CAD build for the part. Positions are in the model's coordinates, mm. Face numbers are marked on the shaded views. Round coordinates to 2 decimals unless told otherwise and drop trailing zeros. Order: outer loops, then holes, each group sorted by start corner. A loop starts at its lowest first (then second) coordinate and runs counter-clockwise, first axis right, second up. Notation, with made-up numbers: (-14, 10.5) - (0, 10.5) arc R13 ccw to (0, 16.5) - close; hole circle Ø9 at (-20.75, 36.25). An arc over 180 degrees is marked (long way). Use one line per item in the form item = value. Start each with the question number.
from build123d import *

# Parameters (mm, degrees)
SKETCH_W            = 205
SKETCH_H            = 115
PAD_DEPTH           = 1.5
SKETCH001_W         = 205
SKETCH001_H         = 115
SKETCH001_W_2       = 200
SKETCH001_H_2       = 110
PAD001_DEPTH        = 7
SKETCH004_W         = 20.8
SKETCH004_H         = 1.2
POCKET_DEPTH        = 1.501
POCKET_DEPTH_BACK   = 7.001
POCKET001_DEPTH     = 10.4
PAD007_DEPTH        = 28.857143
LINEARPATTERN_COUNT = 4
LINEARPATTERN_PITCH = 58.714286
FILLET_R            = 2
CHAMFER_SIZE        = 1


with BuildPart() as part:
    # Sketch → Pad (new body)
    with BuildSketch(Plane.XY):
        Rectangle(SKETCH_W, SKETCH_H)
    extrude(amount=-PAD_DEPTH)

    # Sketch001 → Pad001 (join)
    with BuildSketch(Plane.XY):
        Rectangle(SKETCH001_W, SKETCH001_H)
        Rectangle(SKETCH001_W_2, SKETCH001_H_2, mode=Mode.SUBTRACT)
    extrude(amount=PAD001_DEPTH)

    # Sketch004 → Pocket (cut, two sides)
    with BuildSketch(Plane.XY) as pocket_sk:
        with Locations((0, -56.9)):
            Rectangle(SKETCH004_W, SKETCH004_H)
    extrude(amount=-POCKET_DEPTH, mode=Mode.SUBTRACT)
    extrude(pocket_sk.sketch, amount=POCKET_DEPTH_BACK, mode=Mode.SUBTRACT)

    # Sketch005 → Pocket001 (cut, symmetric)
    with BuildSketch(Plane.YZ):
        Polygon((-56.3, -1.5), (-55.3, -0.6609), (-55.3, 0.3391), (-56.3, 1.178199), align=None)
    extrude(amount=POCKET001_DEPTH, both=True, mode=Mode.SUBTRACT)

    # Sketch008 → Pad007 (join)
    with BuildSketch(Plane.YZ.offset(-102.5)):
        with BuildLine():
            Line((57.5, 7), (57.8, 7.3))
            ThreePointArc((61.906969, 5.384889), (61.356546, 9.565769), (57.8, 7.3))
            Line((61.906969, 5.384889), (57.5, 1.687003))
            Line((57.5, 7), (57.5, 1.687003))
        make_face()
        with BuildLine():
            Line((59.41611, 8.183877), (60.3, 9.067767))
            Line((60.3, 9.067767), (61.183875, 8.183892))
            ThreePointArc((59.41611, 8.183877), (60.30001, 6.05), (61.183875, 8.183892))
        make_face(mode=Mode.SUBTRACT)
    pad007 = extrude(amount=PAD007_DEPTH)

    # LinearPattern: Pad007 ×4
    with Locations(*[(i * LINEARPATTERN_PITCH, 0, 0) for i in range(1, LINEARPATTERN_COUNT)]):
        add(pad007)

    # Fillet
    fillet_edges = [part.edges().sort_by_distance(p)[0] for p in [
        (102.5, -57.5, 2.75),
        (102.5, 57.5, 0.093501),
        (-102.5, 57.5, 0.093501),
        (-102.5, -57.5, 2.75),
    ]]
    fillet(fillet_edges, radius=FILLET_R)

    # Chamfer
    chamfer_edges = [part.edges().sort_by_distance(p)[0] for p in [
        (55.45, -57.5, -1.5),
    ]]
    chamfer(chamfer_edges, length=CHAMFER_SIZE)


solid = part.part
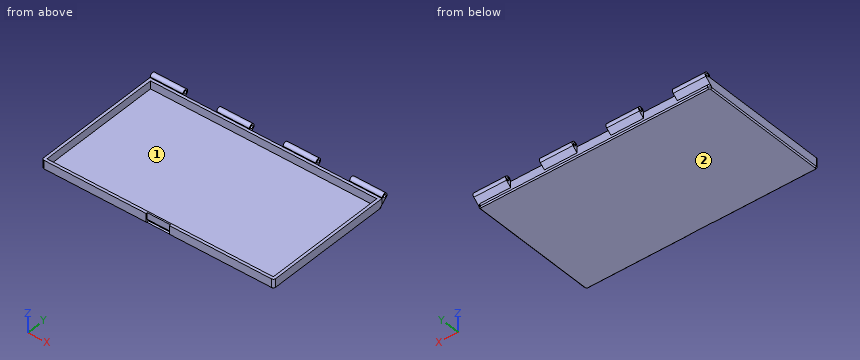
(1) Wall check: line 1 (Y direction, x = 45.5, z = 6); line 2 (X direction, y = 39, z = 3.25); line 3 (Z direction, x = 80.5, y = 54.5). Give the ranges that are in metal, low to high. Write a range as [from, to].
(2) Slice it at A-A (x = -62.5). Give the cut face in (y, z), and give its area (4 significant figures).
(3) Flat gauge pins, fed straight in: P1, Ø5.5, axis at x = 44, z = 2, coming from the +Y side; P2, Ø12, axis at x = 63.5, y = 26.5, coming from the +Z side; P3, Ø1.1, axis at x = 0.5, z = 0, coming from the -Y side. Where does each tip first touch, or does it go through?
(4) Mould opens along X. For the marked faces 1 and 2 say: pulls with the +X half, pulls with the -X half, needs draft (parallel to the pull), parting line crosses it, or undercut.
(5) Slice it at B-B (y = -9.5). Give the cut face in (x, z).
Results list:
q1.line_1 = [-57.5, -55], [55, 57.5]
q1.line_2 = [-102.5, -100], [100, 102.5]
q1.line_3 = [-1.5, 0]
q2.outline = (-57.5, -0.5) - (-56.5, -1.5) - (56.5, -1.5) - (57.5, -0.5) - (57.5, 7) - (55, 7) - (55, 0) - (-55, 0) - (-55, 7) - (-57.5, 7) - close
q2.area = 206.5 mm²
q3.P1 = 61.14
q3.P2 = 0
q3.P3 = -55.55
q4.face_1 = undercut
q4.face_2 = needs draft
q5.outline = (-102.5, -0.5) - (-101.5, -1.5) - (101.5, -1.5) - (102.5, -0.5) - (102.5, 7) - (100, 7) - (100, 0) - (-100, 0) - (-100, 7) - (-102.5, 7) - close
